```python
from build123d import *

# Parameters (mm, degrees)
SKETCH2_W            = 12
SKETCH2_H            = 37.15
BOSS_EXTRUDE2_DEPTH  = 2.5
SKETCH11_W           = 12
SKETCH11_H           = 4
BOSS_EXTRUDE8_DEPTH  = 30
CUT_EXTRUDE1_DEPTH   = 1.7
SKETCH14_W           = 12
SKETCH14_H           = 37.15
BOSS_EXTRUDE9_DEPTH  = 7.5
SKETCH16_W           = 12
SKETCH16_H           = 4
BOSS_EXTRUDE11_DEPTH = 30
CUT_EXTRUDE4_DEPTH   = 1.7
SKETCH22_R           = 3.6
CUT_EXTRUDE6_DEPTH   = 54.483943136
SKETCH23_R           = 3.6
CUT_EXTRUDE7_DEPTH   = 54.483943136
FILLET1_R            = 5
FILLET2_R            = 5
FILLET3_R            = 5
FILLET4_R            = 5


with BuildPart() as part:
    # Sketch2 → Boss-Extrude2 (new body)
    with BuildSketch(Plane.XY):
        with Locations((-2.61160109, -17.608451256)):
            Rectangle(SKETCH2_W, SKETCH2_H)
    extrude(amount=BOSS_EXTRUDE2_DEPTH)

    # Sketch11 → Boss-Extrude8 (add)
    with BuildSketch(Plane.XY.offset(2.5)):
        with Locations((-2.61160109, -1.033451256)):
            Rectangle(SKETCH11_W, SKETCH11_H)
        with Locations((-2.61160109, -34.183451256)):
            Rectangle(SKETCH11_W, SKETCH11_H)
    extrude(amount=BOSS_EXTRUDE8_DEPTH)

    # Sketch12 → Cut-Extrude1 (cut)
    with BuildSketch(Plane(origin=(0, 0.966548744, 0), x_dir=(1, 0, 0), z_dir=(0, 1, 0))):
        with BuildLine():
            Line((-0.514266567, -13.168774056), (0.08839891, -25.11882382))
            ThreePointArc((0.08839891, -25.11882382), (-2.61160109, -31.1), (-5.31160109, -25.11882382))
            Line((-5.31160109, -25.11882382), (-4.708935612, -13.168774056))
            ThreePointArc((-4.708935612, -13.168774056), (-2.61160109, -11.174546931), (-0.514266567, -13.168774056))
        make_face()
    extrude(amount=-CUT_EXTRUDE1_DEPTH, mode=Mode.SUBTRACT)

    # Sketch14 → Boss-Extrude9 (add)
    with BuildSketch(Plane(origin=(0, 0, 0), x_dir=(-1, 0, 0), z_dir=(0, 0, -1))):
        with Locations((2.61160109, -17.608451256)):
            Rectangle(SKETCH14_W, SKETCH14_H)
    extrude(amount=BOSS_EXTRUDE9_DEPTH)

    # Sketch16 → Boss-Extrude11 (add)
    with BuildSketch(Plane(origin=(0, 0, -7.5), x_dir=(-1, 0, 0), z_dir=(0, 0, -1))):
        with Locations((2.61160109, -1.033451256)):
            Rectangle(SKETCH16_W, SKETCH16_H)
        with Locations((2.61160109, -34.183451256)):
            Rectangle(SKETCH16_W, SKETCH16_H)
    extrude(amount=BOSS_EXTRUDE11_DEPTH)

    # Sketch20 → Cut-Extrude4 (cut)
    with BuildSketch(Plane(origin=(0, 0.966548744, 0), x_dir=(1, 0, 0), z_dir=(0, 1, 0))):
        with BuildLine():
            Line((-4.708935612, 18.168774056), (-5.31160109, 30.11882382))
            ThreePointArc((-5.31160109, 30.11882382), (-2.61160109, 36.1), (0.08839891, 30.11882382))
            Line((0.08839891, 30.11882382), (-0.514266567, 18.168774056))
            ThreePointArc((-0.514266567, 18.168774056), (-2.61160109, 16.174546931), (-4.708935612, 18.168774056))
        make_face()
    extrude(amount=-CUT_EXTRUDE4_DEPTH, mode=Mode.SUBTRACT)

    # Sketch22 → Cut-Extrude6 (cut, through all)
    with BuildSketch(Plane(origin=(0, 0.966548744, 0), x_dir=(1, 0, 0), z_dir=(0, 1, 0))):
        with Locations(Location((-2.61160109, -27.5, 0), (0, 0, 270))):
            Circle(SKETCH22_R)
    extrude(amount=-CUT_EXTRUDE6_DEPTH, mode=Mode.SUBTRACT)

    # Sketch23 → Cut-Extrude7 (cut, through all)
    with BuildSketch(Plane(origin=(0, 0.966548744, 0), x_dir=(1, 0, 0), z_dir=(0, 1, 0))):
        with Locations(Location((-2.61160109, 32.5, 0), (0, 0, 221.409622109))):
            Circle(SKETCH23_R)
    extrude(amount=-CUT_EXTRUDE7_DEPTH, mode=Mode.SUBTRACT)

    # Fillet1
    fillet1_edges = [part.edges().sort_by_distance(p)[0] for p in [
        (-2.61160109, -3.033451256, 2.5),
    ]]
    fillet(fillet1_edges, radius=FILLET1_R)

    # Fillet2
    fillet2_edges = [part.edges().sort_by_distance(p)[0] for p in [
        (-2.61160109, -32.183451256, 2.5),
    ]]
    fillet(fillet2_edges, radius=FILLET2_R)

    # Fillet3
    fillet3_edges = [part.edges().sort_by_distance(p)[0] for p in [
        (-2.61160109, -3.033451256, -7.5),
    ]]
    fillet(fillet3_edges, radius=FILLET3_R)

    # Fillet4
    fillet4_edges = [part.edges().sort_by_distance(p)[0] for p in [
        (-2.61160109, -32.183451256, -7.5),
    ]]
    fillet(fillet4_edges, radius=FILLET4_R)


solid = part.part
```
Could you check a few things on this model? Use its own coordinates, in mm. A direction names the side the tool comes from. Round coordinates to 2 decimals unless told otherwise and drop trailing zeros. Write each loop counter-clockwise with the first axis right and the second up, starting at its lowest first coordinate (ties: lowest second). Pieces come first, ordered by that corner, then holes. Notation, with made-up numbers: M 42,-9 L 101,-9 A20 ccw 101,30 Z; hole C -11.75,27.25 d4. An arc over 180 degrees is marked long. Answer in a Markdown table with one row per item. Add a question column.
Q1. If I drill on line 1 (Y direction, x = -5, z = 17); line 2 (X direction, y = -1.75, z = 27.5); line 3 (Y direction, x = -4, z = 21.5), over which ranges is the centre line in solid material (lowest first)? Write a range as from..to.
Q2. Imagine slicing it at C-C (z = 4). Please give me the cut outline in (x, y).
Q3. Imagine slicing it at A-A (z = -32.5). Please give me the cut outline in (x, y).
Q4. Imagine slicing it at D-D (y = -11). Please give me the cut outline in (x, z).
Q5. Will these pins go through, and if not, where does the flat tip stop? pin 1 Ø6 at (x, y) = (-1.5, -19.5) entering from -Z; pin 2 Ø10 at (y, z) = (-23, -15.5) entering from +X; pin 3 Ø3 at (x, y) = (2, -29.5) entering from +Z.
Q6. Imagine slicing it at B-B (y = -2). Please give me the cut outline in (x, z), then the cut area to 3 significant figures.
Q7. If we mould it in two halves opening along X, with no side actions, what happens to faces 1 (the flat face through (3.388, -16, -2)), 2 (the flat face through (-3, -0.733, -23)), 3 (the flat face through (-3, -34, 32.5)), 4 (the flat face through (-8.612, -16, -2))? For each: +X half, -X half, draft (parallel to the pull), parting line (faces both ways), or undercut.
Q8. On a 3-axis mill with a long thin cutter (end or side, diameter ignored), from which of +Z, -Z, +X, -X, +Y, -Y can I reach the whole of each face in a straight line? I mean faces 5 (the flat face through (-3, 0.967, -2)), 6 (the cylindrical face through (-2.528, -30.68, 3.926)), 7 (the cylindrical face through (-2.567, 0.128, -16.175)), 8 (the cylindrical face through (-2.696, -30.68, -8.926)). Say none if no direction works.
Values:
| question | item | result |
|---|---|---|
| 1 | line 1 | -36.18..-32.18, -3.03..0.97 |
| 1 | line 2 | -8.61..-6.21, 0.99..3.39 |
| 1 | line 3 | -36.18..-32.18, -3.03..-0.73 |
| 2 | outline | M -8.61,-36.18 L 3.39,-36.18 L 3.39,-30.75 L -8.61,-30.75 Z; M -8.61,-4.46 L 3.39,-4.46 L 3.39,0.97 L -8.61,0.97 Z |
| 3 | outline | M -8.61,-36.18 L -6.21,-36.18 L -6.21,-32.18 L -8.61,-32.18 Z; M -8.61,-3.03 L -6.21,-3.03 L -6.21,0.97 L -8.61,0.97 Z; M 0.99,-36.18 L 3.39,-36.18 L 3.39,-32.18 L 0.99,-32.18 Z; M 0.99,-3.03 L 3.39,-3.03 L 3.39,0.97 L 0.99,0.97 Z |
| 4 | outline | M -8.61,-7.5 L 3.39,-7.5 L 3.39,2.5 L -8.61,2.5 Z |
| 5 | pin 1 | z = -7.5 |
| 5 | pin 2 | through |
| 5 | pin 3 | z = 4.27 |
| 6 | outline | M -8.61,-37.5 L 3.39,-37.5 L 3.39,32.5 L -8.61,32.5 Z; hole C -2.61,-32.5 d7.2; hole C -2.61,27.5 d7.2 |
| 6 | area | 759 mm^2 |
| 7 | face 1 | +X half |
| 7 | face 2 | undercut |
| 7 | face 3 | draft |
| 7 | face 4 | -X half |
| 8 | face 5 | +Z, -Z, +X, -X, +Y |
| 8 | face 6 | +Z, +X, -X |
| 8 | face 7 | +Y |
| 8 | face 8 | -Z, +X, -X |
